from build123d import *

# Parameters (mm, degrees)
SKETCH1_R           = 2.1
BOSS_EXTRUDE1_DEPTH = 80


with BuildPart() as part:
    # Sketch1 → Boss-Extrude1 (new body)
    with BuildSketch(Plane.XY.offset(500)):
        with BuildLine():
            Line((6.560660172, 14.5), (3.9, 17.160660172))
            Line((3.9, 17.160660172), (3.9, 19.79))
            Line((3.9, 19.79), (3.69, 20))
            Line((3.69, 20), (3.9, 20.21))
            Line((3.9, 20.21), (3.9, 22.839339828))
            Line((3.9, 22.839339828), (6.560660172, 25.5))
            Line((6.560660172, 25.5), (8.2, 25.5))
            Line((8.2, 25.5), (8.2, 23.125))
            Line((8.2, 23.125), (8.545, 23.125))
            Line((8.545, 23.125), (10, 24.58))
            Line((10, 24.58), (10, 29.5))
            ThreePointArc((10, 29.5), (9.853553391, 29.853553391), (9.5, 30))
            Line((9.5, 30), (4.58, 30))
            Line((4.58, 30), (3.125, 28.545))
            Line((3.125, 28.545), (3.125, 28.2))
            Line((3.125, 28.2), (5.5, 28.2))
            Line((5.5, 28.2), (5.5, 26.560660172))
            Line((5.5, 26.560660172), (2.839339828, 23.9))
            Line((2.839339828, 23.9), (0.21, 23.9))
            Line((0.21, 23.9), (0, 23.69))
            Line((0, 23.69), (-0.21, 23.9))
            Line((-0.21, 23.9), (-2.839339828, 23.9))
            Line((-2.839339828, 23.9), (-5.5, 26.560660172))
            Line((-5.5, 26.560660172), (-5.5, 28.2))
            Line((-5.5, 28.2), (-3.125, 28.2))
            Line((-3.125, 28.2), (-3.125, 28.545))
            Line((-3.125, 28.545), (-4.58, 30))
            Line((-4.58, 30), (-9.5, 30))
            ThreePointArc((-9.5, 30), (-9.853553391, 29.853553391), (-10, 29.5))
            Line((-10, 29.5), (-10, 24.58))
            Line((-10, 24.58), (-8.545, 23.125))
            Line((-8.545, 23.125), (-8.2, 23.125))
            Line((-8.2, 23.125), (-8.2, 25.5))
            Line((-8.2, 25.5), (-6.560660172, 25.5))
            Line((-6.560660172, 25.5), (-3.9, 22.839339828))
            Line((-3.9, 22.839339828), (-3.9, 20.21))
            Line((-3.9, 20.21), (-3.69, 20))
            Line((-3.69, 20), (-3.9, 19.79))
            Line((-3.9, 19.79), (-3.9, 17.160660172))
            Line((-3.9, 17.160660172), (-6.560660172, 14.5))
            Line((-6.560660172, 14.5), (-8.2, 14.5))
            Line((-8.2, 14.5), (-8.2, 16.875))
            Line((-8.2, 16.875), (-8.545, 16.875))
            Line((-8.545, 16.875), (-10, 15.42))
            Line((-10, 15.42), (-10, 4.58))
            Line((-10, 4.58), (-8.545, 3.125))
            Line((-8.545, 3.125), (-8.2, 3.125))
            Line((-8.2, 3.125), (-8.2, 5.5))
            Line((-8.2, 5.5), (-6.560660172, 5.5))
            Line((-6.560660172, 5.5), (-3.9, 2.839339828))
            Line((-3.9, 2.839339828), (-3.9, 0.21))
            Line((-3.9, 0.21), (-3.69, 0))
            Line((-3.69, 0), (-3.9, -0.21))
            Line((-3.9, -0.21), (-3.9, -2.839339828))
            Line((-3.9, -2.839339828), (-6.560660172, -5.5))
            Line((-6.560660172, -5.5), (-8.2, -5.5))
            Line((-8.2, -5.5), (-8.2, -3.125))
            Line((-8.2, -3.125), (-8.545, -3.125))
            Line((-8.545, -3.125), (-10, -4.58))
            Line((-10, -4.58), (-10, -15.42))
            Line((-10, -15.42), (-8.545, -16.875))
            Line((-8.545, -16.875), (-8.2, -16.875))
            Line((-8.2, -16.875), (-8.2, -14.5))
            Line((-8.2, -14.5), (-6.560660172, -14.5))
            Line((-6.560660172, -14.5), (-3.9, -17.160660172))
            Line((-3.9, -17.160660172), (-3.9, -19.79))
            Line((-3.9, -19.79), (-3.69, -20))
            Line((-3.69, -20), (-3.9, -20.21))
            Line((-3.9, -20.21), (-3.9, -22.839339828))
            Line((-3.9, -22.839339828), (-6.560660172, -25.5))
            Line((-6.560660172, -25.5), (-8.2, -25.5))
            Line((-8.2, -25.5), (-8.2, -23.125))
            Line((-8.2, -23.125), (-8.545, -23.125))
            Line((-8.545, -23.125), (-10, -24.58))
            Line((-10, -24.58), (-10, -29.5))
            ThreePointArc((-10, -29.5), (-9.853553391, -29.853553391), (-9.5, -30))
            Line((-9.5, -30), (-4.58, -30))
            Line((-4.58, -30), (-3.125, -28.545))
            Line((-3.125, -28.545), (-3.125, -28.2))
            Line((-3.125, -28.2), (-5.5, -28.2))
            Line((-5.5, -28.2), (-5.5, -26.560660172))
            Line((-5.5, -26.560660172), (-2.839339828, -23.9))
            Line((-2.839339828, -23.9), (-0.21, -23.9))
            Line((-0.21, -23.9), (0, -23.69))
            Line((0, -23.69), (0.21, -23.9))
            Line((0.21, -23.9), (2.839339828, -23.9))
            Line((2.839339828, -23.9), (5.5, -26.560660172))
            Line((5.5, -26.560660172), (5.5, -28.2))
            Line((5.5, -28.2), (3.125, -28.2))
            Line((3.125, -28.2), (3.125, -28.545))
            Line((3.125, -28.545), (4.58, -30))
            Line((4.58, -30), (9.5, -30))
            ThreePointArc((9.5, -30), (9.853553391, -29.853553391), (10, -29.5))
            Line((10, -29.5), (10, -24.58))
            Line((10, -24.58), (8.545, -23.125))
            Line((8.545, -23.125), (8.2, -23.125))
            Line((8.2, -23.125), (8.2, -25.5))
            Line((8.2, -25.5), (6.560660172, -25.5))
            Line((6.560660172, -25.5), (3.9, -22.839339828))
            Line((3.9, -22.839339828), (3.9, -20.21))
            Line((3.9, -20.21), (3.69, -20))
            Line((3.69, -20), (3.9, -19.79))
            Line((3.9, -19.79), (3.9, -17.160660172))
            Line((3.9, -17.160660172), (6.560660172, -14.5))
            Line((6.560660172, -14.5), (8.2, -14.5))
            Line((8.2, -14.5), (8.2, -16.875))
            Line((8.2, -16.875), (8.545, -16.875))
            Line((8.545, -16.875), (10, -15.42))
            Line((10, -15.42), (10, -4.58))
            Line((10, -4.58), (8.545, -3.125))
            Line((8.545, -3.125), (8.2, -3.125))
            Line((8.2, -3.125), (8.2, -5.5))
            Line((8.2, -5.5), (6.560660172, -5.5))
            Line((6.560660172, -5.5), (3.9, -2.839339828))
            Line((3.9, -2.839339828), (3.9, -0.21))
            Line((3.9, -0.21), (3.69, 0))
            Line((3.69, 0), (3.9, 0.21))
            Line((3.9, 0.21), (3.9, 2.839339828))
            Line((3.9, 2.839339828), (6.560660172, 5.5))
            Line((6.560660172, 5.5), (8.2, 5.5))
            Line((8.2, 5.5), (8.2, 3.125))
            Line((8.2, 3.125), (8.545, 3.125))
            Line((8.545, 3.125), (10, 4.58))
            Line((10, 4.58), (10, 15.42))
            Line((10, 15.42), (8.545, 16.875))
            Line((8.545, 16.875), (8.2, 16.875))
            Line((8.2, 16.875), (8.2, 14.5))
            Line((8.2, 14.5), (6.560660172, 14.5))
        make_face()
        with Locations(Location((0, 20, 0), (0, 0, 180))):
            Circle(SKETCH1_R, mode=Mode.SUBTRACT)
        with Locations(Location((0, 0, 0), (0, 0, 180))):
            Circle(SKETCH1_R, mode=Mode.SUBTRACT)
        with Locations(Location((0, -20, 0), (0, 0, 180))):
            Circle(SKETCH1_R, mode=Mode.SUBTRACT)
        Polygon((2.839339828, 3.9), (-2.839339828, 3.9), (-6.239339828, 7.3), (-8.2, 7.3), (-8.2, 12.7), (-6.239339828, 12.7), (-2.839339828, 16.1), (2.839339828, 16.1), (6.239339828, 12.7), (8.2, 12.7), (8.2, 7.3), (6.239339828, 7.3), align=None, mode=Mode.SUBTRACT)
        Polygon((2.839339828, -16.1), (-2.839339828, -16.1), (-6.239339828, -12.7), (-8.2, -12.7), (-8.2, -7.3), (-6.239339828, -7.3), (-2.839339828, -3.9), (2.839339828, -3.9), (6.239339828, -7.3), (8.2, -7.3), (8.2, -12.7), (6.239339828, -12.7), align=None, mode=Mode.SUBTRACT)
    extrude(amount=-BOSS_EXTRUDE1_DEPTH)


solid = part.part
Part model, mm, in its own coordinate system. A direction names the side the tool comes from. Coordinates: 2 decimals unless noted, no trailing zeros. Use a Markdown table: item, result.
(1) Tool access for faces 1 (the flat face through (-10, -27, 461)), 2 (the flat face through (-3.9, 22, 461)), 3 (the flat face through (7, 12.7, 461)): list every direction of +Z, -Z, +X, -X, +Y, -Y with a clear straight run to the whole face (end or side of a thin tool).
A:
| item | result |
|---|---|
| face 1 | +Z, -Z, -X, +Y, -Y |
| face 2 | +Z, -Z, -X |
| face 3 | +Z, -Z |
(2) Cut at A-A on z = 443.5. State how many separate pieces and enclosed holes the cut face has, then the cut area to 3 significant figures.
A:
| item | result |
|---|---|
| separate pieces | 1 |
| enclosed holes | 5 |
| area | 429 mm^2 |
(3) Probe L1, parallel to Y at x = 0, z = 443.5; L2, parallel to Y at x = 8, z = 479; L3, parallel to Y at x = 2.75, z = 469. List the from-to ranges inside material, lowest first.
A:
| item | result |
|---|---|
| L1 | y = -23.69 to -22.1, -17.9 to -16.1, -3.9 to -2.1, 2.1 to 3.9, 16.1 to 17.9, 22.1 to 23.69 |
| L2 | y = -30 to -25.5, -14.5 to -12.7, -7.3 to -5.5, 5.5 to 7.3, 12.7 to 14.5, 25.5 to 30 |
| L3 | y = -23.9 to -16.1, -3.9 to 3.9, 16.1 to 23.9 |
(4) Pull direction Y, two halves, no side cores. Call faces 4 (the flat face through (-7, -30, 461)), 5 (the flat face through (2, 23.9, 461)), 6 (the flat face through (-4.19, -25.25, 460.56)): released by +Y, released by -Y, zero draft, split by the parting line, or undercut.
A:
| item | result |
|---|---|
| face 4 | released by -Y |
| face 5 | released by +Y |
| face 6 | undercut |
(5) Flat gauge pins, fed straight in: pin 1 (1.9 mm diameter, centred on y = -4.5, z = 462.5, fed in from -X); pin 2 (5 mm diameter, centred on y = 0.5, z = 451.5, fed in from -X); pin 3 (1.7 mm diameter, centred on x = -0.5, z = 468.5, fed in from -Y); pin 4 (1 mm diameter, centred on x = -0.5, y = -19.5, fed in from +Z). Where does each tip first touch, or does it go through?
A:
| item | result |
|---|---|
| pin 1 | stops at x = -10 |
| pin 2 | stops at x = -4.06 |
| pin 3 | stops at y = -23.9 |
| pin 4 | passes through |
